The listing builds one solid part. Answer for the finished solid, in the listing's coordinates (mm). A direction names the side the tool comes from. Coordinates: 2 decimals unless noted, no trailing zeros. Loops run counter-clockwise (first coordinate to the right, second up) from the corner with the lowest first, then second, coordinate; pieces in that order, holes last. Notation, with made-up numbers: M -13.75,85 L -0.75,85 A15 ccw -0.75,91 Z; hole C 49,-1 d8. An arc over 180 degrees is marked long. Return JSON: item names as keys, results as strings. Group by question number.
1. Section B-B (z = -1.5) is taken. Write down the section's boundary in (x, y), then the cut area to 3 significant figures.
2. Straight lines are drawn through the part: L1, parallel to X at y = 16.5, z = 4; L2, parallel to Y at x = 13.5, z = 0.5; L3, parallel to Y at x = -4.5, z = 5. For each, find the intervals that lie inside material, in ascending order. Write a range as from..to.
3. Section D-D (z = 3) is taken. Write down the section's boundary in (x, y).
4. Section C-C (x = 10) is taken. Write down the section's boundary in (y, z).
5. Which of the six approach directions +Z, -Z, +X, -X, +Y, -Y give full straight-line access (tool end or side, diameter ignored) to faces 5 (the face through (13.712, 0.507, -1.003)), 6 (the face through (-15, 18, 8.562)), 7 (the face through (-15, 17.6, 2)), 8 (the face through (-14.568, 18.107, 2.515)), 9 (the face through (5.9, 0.3, 8.562))?
6. Section A-A (y = 11.5) is taken. Write down the section's boundary in (x, z), then the cut area to 3 significant figures.
7. Given P1, Ø3, axis at x = -12.5, y = 3.5, coming from the +Z side; P2, Ø0.8, axis at x = -14, y = 18, coming from the +Z side; P3, Ø2.5, axis at x = -14.82, z = -0.94, coming from the -Y side, each flat-ended and moving along its own axis, determine where each tip first touches the part or whether it passes through.
8. The mould has two halves that part along X. Classify faces 1 (the face through (-16.288, 0.507, 5.997)), 2 (the face through (-18.319, 9, 3)), 3 (the face through (-18, 9, 8.615)), 4 (the face through (-17.319, 9, 3)): pulls with the +X half, pulls with the -X half, needs draft (parallel to the pull), parting line crosses it, or undercut.
```python
from build123d import *

# Parameters (mm, degrees)
SKETCH1_W           = 35
SKETCH1_H           = 12
BOSS_EXTRUDE1_DEPTH = 1
SKETCH2_W           = 12.053455819
SKETCH2_H           = 17.6
BOSS_EXTRUDE2_DEPTH = 1
SKETCH3_W           = 12
SKETCH3_H           = 17.6
BOSS_EXTRUDE3_DEPTH = 1
SKETCH5_W           = 37
SKETCH5_H           = 12
BOSS_EXTRUDE4_DEPTH = 1
SKETCH6_W           = 24.58
SKETCH6_H           = 12
CUT_EXTRUDE1_DEPTH  = 1
SKETCH7_R           = 1
CUT_EXTRUDE2_DEPTH  = 1
SKETCH8_R           = 1
CUT_EXTRUDE3_DEPTH  = 1
SKETCH9_R           = 1.47
CUT_EXTRUDE4_DEPTH  = 10


with BuildPart() as part:
    # Sketch1 → Boss-Extrude1 (new body)
    with BuildSketch(Plane(origin=(0, 0, 0), x_dir=(1, 0, 0), z_dir=(0, 1, 0))):
        with Locations((0.180945347, -2.562038405)):
            Rectangle(SKETCH1_W, SKETCH1_H)
    extrude(amount=BOSS_EXTRUDE1_DEPTH)

    # Sketch2 → Boss-Extrude2 (add)
    with BuildSketch(Plane.ZY.offset(17.319054653)):
        with Locations((2.588766314, 8.8)):
            Rectangle(SKETCH2_W, SKETCH2_H)
    extrude(amount=BOSS_EXTRUDE2_DEPTH)

    # Sketch3 → Boss-Extrude3 (add)
    with BuildSketch(Plane(origin=(17.680945347, 0, 0), x_dir=(0, 0, -1), z_dir=(1, 0, 0))):
        with Locations((-2.562038405, 8.8)):
            Rectangle(SKETCH3_W, SKETCH3_H)
    extrude(amount=BOSS_EXTRUDE3_DEPTH)

    # Sketch5 → Boss-Extrude4 (add)
    with BuildSketch(Plane(origin=(0, 17.6, 0), x_dir=(1, 0, 0), z_dir=(0, 1, 0))):
        with Locations((0.180945347, -2.562038405)):
            Rectangle(SKETCH5_W, SKETCH5_H)
    extrude(amount=BOSS_EXTRUDE4_DEPTH)

    # Sketch6 → Cut-Extrude1 (cut)
    with BuildSketch(Plane(origin=(0, 18.6, 0), x_dir=(1, 0, 0), z_dir=(0, 1, 0))):
        with Locations((0.180945347, -2.562038405)):
            Rectangle(SKETCH6_W, SKETCH6_H)
    extrude(amount=-CUT_EXTRUDE1_DEPTH, mode=Mode.SUBTRACT)

    # Sketch7 → Cut-Extrude2 (cut)
    with BuildSketch(Plane(origin=(0, 18.6, 0), x_dir=(1, 0, 0), z_dir=(0, 1, 0))):
        with Locations((13.680945347, -2.562038405)):
            Circle(SKETCH7_R)
    extrude(amount=-CUT_EXTRUDE2_DEPTH, mode=Mode.SUBTRACT)

    # Sketch8 → Cut-Extrude3 (cut)
    with BuildSketch(Plane(origin=(0, 18.6, 0), x_dir=(1, 0, 0), z_dir=(0, 1, 0))):
        with Locations((-13.569054453, -2.558738176)):
            Circle(SKETCH8_R)
    extrude(amount=-CUT_EXTRUDE3_DEPTH, mode=Mode.SUBTRACT)

    # Sketch9 → Cut-Extrude4 (cut)
    with BuildSketch(Plane(origin=(0, 1, 0), x_dir=(1, 0, 0), z_dir=(0, 1, 0))):
        with Locations((15.180945347, 0.937961595)):
            Circle(SKETCH9_R)
        with Locations((15.180945347, -6.062038405)):
            Circle(SKETCH9_R)
        with Locations((-14.819054653, 0.937961595)):
            Circle(SKETCH9_R)
        with Locations((-14.819054653, -6.062038405)):
            Circle(SKETCH9_R)
    extrude(amount=-CUT_EXTRUDE4_DEPTH, mode=Mode.SUBTRACT)


solid = part.part
```
Worked out:
{
 "1": {"outline": "M -18.32,0 L -16.18,0 L -16.18,1 L -17.32,1 L -17.32,17.6 L -12.11,17.6 L -12.11,18.6 L -18.32,18.6 Z; M -13.46,0 L 13.82,0 L 13.82,1 L -13.46,1 Z; M 12.47,17.6 L 17.68,17.6 L 17.68,1 L 16.54,1 L 16.54,0 L 18.68,0 L 18.68,18.6 L 12.47,18.6 Z", "area": "77.2 mm^2"},
 "2": {"L1": "-18.32..-17.32, 17.68..18.68", "L2": "0..1, 17.6..18.6", "L3": "0..1"},
 "3": {"outline": "M -18.32,0 L 18.68,0 L 18.68,18.6 L 14.58,18.6 L 14.58,17.6 L 17.68,17.6 L 17.68,1 L -17.32,1 L -17.32,17.6 L -14.47,17.6 L -14.47,18.6 L -18.32,18.6 Z; M -12.67,17.6 L -12.11,17.6 L -12.11,18.6 L -12.67,18.6 Z; M 12.47,17.6 L 12.78,17.6 L 12.78,18.6 L 12.47,18.6 Z"},
 "4": {"outline": "M 0,-3.44 L 1,-3.44 L 1,8.56 L 0,8.56 Z"},
 "5": {"face 5": "-Y", "face 6": "+Z, +X, -X, +Y", "face 7": "+Z, -Z", "face 8": "+Y", "face 9": "+Z, +X, +Y, -Y"},
 "6": {"outline": "M -18.32,-3.44 L -17.32,-3.44 L -17.32,8.62 L -18.32,8.62 Z; M 17.68,-3.44 L 18.68,-3.44 L 18.68,8.56 L 17.68,8.56 Z", "area": "24.1 mm^2"},
 "7": {"P1": "through", "P2": "z = 8.56", "P3": "y = 17.6"},
 "8": {"face 1": "undercut", "face 2": "pulls with the -X half", "face 3": "needs draft", "face 4": "undercut"}
}
